Part model, mm, in its own coordinate system. A direction names the side the tool comes from. Coordinates: 2 decimals unless noted, no trailing zeros. Loops run counter-clockwise (first coordinate to the right, second up) from the corner with the lowest first, then second, coordinate; pieces in that order, holes last. Notation, with made-up numbers: M -19.5,66 L 12.5,66 A27 ccw 12.5,88 Z; hole C 72,52 d2. An arc over 180 degrees is marked long. Answer as a JSON object with one key per item and string values. Group by question number.
1. 3-axis set-ups, long thin cutter, end or side, ignore diameter. For faces 1 (the face through (11.5, 2, 0.2)), 2 (the face through (5, 15, 7)), 3 (the face through (0.683, 2, 7)), 4 (the face through (10.7, 2, 13.6)): which of +Z, -Z, +X, -X, +Y, -Y reach the whole face in a straight line?
2. Saw through at A-A on x = 12. Write the cut outline in (y, z), then the cut area to 3 significant figures.
3. Mould opens along Z. For faces 5 (the face through (4, 10, 0)), 6 (the face through (10.7, 3, 13.6)), 7 (the face through (8, 4, 7)) say: released by +Z, released by -Z, zero draft, split by the parting line, or undercut.
4. Saw through at B-B on z = 6.5. Write the cut outline in (x, y).
5. Drop flat-ended pins along their axis: pin 1 Ø4 at (y, z) = (22, 4) entering from +X; pin 2 Ø1.2 at (x, z) = (8, 11.5) entering from -Y; pin 3 Ø3 at (x, z) = (8, 1) entering from +Y. Give the stop position or say it passes through.
6. Drill centre lines: L1, parallel to X at y = 1.5, z = 8; L2, parallel to X at y = 24, z = 11; L3, parallel to Y at x = 6.5, z = 13. Where is each one in solid material? Low to high.
7. Saw through at C-C on x = 1.75. Write the cut outline in (y, z).
8. Saw through at D-D on y = 20. Write the cut outline in (x, z).
from build123d import *

# Parameters (mm, degrees)
BOSS_EXTRUDE3_DEPTH = 14
SKETCH3_W           = 13.981436564
SKETCH3_H           = 12.786132402
CUT_EXTRUDE2_DEPTH  = 4
SKETCH4_W           = 10
SKETCH4_H           = 1
CUT_EXTRUDE3_DEPTH  = 4
SKETCH5_W           = 8
SKETCH5_H           = 1
CUT_EXTRUDE4_DEPTH  = 4
SKETCH6_W           = 1.942983733
SKETCH6_H           = 1
CUT_EXTRUDE5_DEPTH  = 4


with BuildPart() as part:
    # Sketch1 → Boss-Extrude3 (new body)
    with BuildSketch(Plane.XY):
        with BuildLine():
            Line((0, 24), (0, 0))
            Line((0, 0), (15, 0))
            ThreePointArc((15, 0), (15.707106781, 0.292893219), (16, 1))
            Line((16, 1), (16, 4))
            ThreePointArc((16, 4), (15.707106781, 4.707106781), (15, 5))
            Line((15, 5), (6, 5))
            ThreePointArc((6, 5), (5.292893219, 5.292893219), (5, 6))
            Line((5, 6), (5, 24))
            ThreePointArc((5, 24), (4.707106781, 24.707106781), (4, 25))
            Line((4, 25), (1, 25))
            ThreePointArc((1, 25), (0.292893219, 24.707106781), (0, 24))
        make_face()
    extrude(amount=BOSS_EXTRUDE3_DEPTH)

    # Sketch3 → Cut-Extrude2 (cut)
    with BuildSketch(Plane.XZ):
        with Locations((7.674007956, 6.864169982)):
            Rectangle(SKETCH3_W, SKETCH3_H)
    extrude(amount=-CUT_EXTRUDE2_DEPTH, mode=Mode.SUBTRACT)

    # Sketch4 → Cut-Extrude3 (cut)
    with BuildSketch(Plane.XY.offset(14)):
        with Locations((10, 2.5)):
            Rectangle(SKETCH4_W, SKETCH4_H)
    extrude(amount=-CUT_EXTRUDE3_DEPTH, mode=Mode.SUBTRACT)

    # Sketch5 → Cut-Extrude4 (cut)
    with BuildSketch(Plane(origin=(0, 0, 0), x_dir=(-1, 0, 0), z_dir=(0, 0, -1))):
        with Locations((-11, 2.5)):
            Rectangle(SKETCH5_W, SKETCH5_H)
    extrude(amount=-CUT_EXTRUDE4_DEPTH, mode=Mode.SUBTRACT)

    # Sketch6 → Cut-Extrude5 (cut)
    with BuildSketch(Plane(origin=(0, 0, 0), x_dir=(-1, 0, 0), z_dir=(0, 0, -1))):
        with Locations((-6.028508134, 2.5)):
            Rectangle(SKETCH6_W, SKETCH6_H)
    extrude(amount=-CUT_EXTRUDE5_DEPTH, mode=Mode.SUBTRACT)


solid = part.part
Outcome:
{
 "1": {"face 1": "-Z", "face 2": "+Z, -Z, +X, +Y", "face 3": "-Y", "face 4": "+Z"},
 "2": {"outline": "M 0,0 L 2,0 L 2,0.47 L 0,0.47 Z; M 0,13.26 L 2,13.26 L 2,14 L 0,14 Z; M 3,0 L 5,0 L 5,14 L 3,14 L 3,13.26 L 4,13.26 L 4,0.47 L 3,0.47 Z", "area": "17.6 mm²"},
 "3": {"face 5": "released by -Z", "face 6": "zero draft", "face 7": "undercut"},
 "4": {"outline": "M 0,0 L 0.68,0 L 0.68,4 L 14.66,4 L 14.66,0 L 15,0 A1 ccw 16,1 L 16,4 A1 ccw 15,5 L 6,5 A1 cw 5,6 L 5,24 A1 ccw 4,25 L 1,25 A1 ccw 0,24 Z"},
 "5": {"pin 1": "stops at x = 5", "pin 2": "stops at y = 4", "pin 3": "stops at y = 5"},
 "6": {"L1": "x = 0 to 0.68, 14.66 to 16", "L2": "x = 0 to 5", "L3": "y = 4 to 5"},
 "7": {"outline": "M 0,0 L 25,0 L 25,14 L 0,14 L 0,13.26 L 4,13.26 L 4,0.47 L 0,0.47 Z"},
 "8": {"outline": "M 0,0 L 5,0 L 5,14 L 0,14 Z"}
}
